```python
from build123d import *

# Parameters (mm, degrees)
SKETCH1_R           = 48.26
SKETCH1_R_2         = 26.56205
SKETCH1_W           = 81.370000074
SKETCH1_H           = 40
BOSS_EXTRUDE2_DEPTH = 15.24
SKETCH2_W           = 15.24
SKETCH2_H           = 24.76
BOSS_EXTRUDE3_DEPTH = 40
SKETCH3_R           = 3.9773733
SKETCH3_R_2         = 3.985133
CUT_EXTRUDE1_DEPTH  = 170.12215531
FILLET1_R           = 5.08
BOSS_EXTRUDE4_DEPTH = 66.04


with BuildPart() as part:
    # Sketch1 → Boss-Extrude2 (new body)
    # profile 1 of 2: a face of its own
    with BuildSketch(Plane(origin=(0, 0, 0), x_dir=(1, 0, 0), z_dir=(0, 1, 0))):
        Circle(SKETCH1_R)
        with Locations(Location((0, 0, 0), (0, 0, 90))):
            Circle(SKETCH1_R_2, mode=Mode.SUBTRACT)
    # profile 2 of 2: a face of its own
    with BuildSketch(Plane(origin=(0, 0, 0), x_dir=(1, 0, 0), z_dir=(0, 1, 0))):
        with Locations((83.372292456, 2.512722314)):
            Rectangle(SKETCH1_W, SKETCH1_H)
    extrude(amount=BOSS_EXTRUDE2_DEPTH)

    # Sketch2 → Boss-Extrude3 (add)
    with BuildSketch(Plane(origin=(0, 0, -22.512722314), x_dir=(-1, 0, 0), z_dir=(0, 0, -1))):
        with Locations((-116.437292493, 27.62)):
            Rectangle(SKETCH2_W, SKETCH2_H)
    extrude(amount=-BOSS_EXTRUDE3_DEPTH)

    # Sketch3 → Cut-Extrude1 (cut, through all)
    with BuildSketch(Plane.ZY.offset(-108.817292493)):
        with Locations((7.449197686, 31.22176)):
            Circle(SKETCH3_R)
        with Locations((-12.474642314, 31.22176)):
            Circle(SKETCH3_R_2)
    extrude(amount=-CUT_EXTRUDE1_DEPTH, mode=Mode.SUBTRACT)

    # Fillet1
    fillet1_edges = [part.edges().sort_by_distance(p)[0] for p in [
        (108.817292493, 15.24, -2.512722314),
    ]]
    fillet(fillet1_edges, radius=FILLET1_R)

    # Sketch5 → Boss-Extrude4 (add)
    with BuildSketch(Plane(origin=(0, 15.24, 0), x_dir=(1, 0, 0), z_dir=(0, 1, 0))):
        with BuildLine():
            ThreePointArc((0, 39.248127244), (39.248127244, 0), (0, -39.248127244))
            Line((0, -39.248127244), (-28.082238298, -39.248127244))
            ThreePointArc((-28.082238298, -39.248127244), (22.065570237, -42.920137583), (48.26, 0))
            ThreePointArc((48.26, 0), (22.065570237, 42.920137583), (-28.082238298, 39.248127244))
            Line((-28.082238298, 39.248127244), (0, 39.248127244))
        make_face()
    extrude(amount=BOSS_EXTRUDE4_DEPTH)


solid = part.part
```
CAD build for the part. Positions are in the model's coordinates, mm. A direction names the side the tool comes from. Round coordinates to 2 decimals unless told otherwise and drop trailing zeros. Loops run counter-clockwise (first coordinate to the right, second up) from the corner with the lowest first, then second, coordinate; pieces in that order, holes last. Notation, with made-up numbers: (76, 71.25) - (90, 71.25) arc R16 ccw to (90, 77.25) - close; hole circle Ø5 at (39.5, 49.5). An arc over 180 degrees is marked (long way). Return JSON: item names as keys, results as strings. Group by question number.
Q1. Band-saw the part on C-C on y = 50. Give the cut face in (x, z).
Q2. Band-saw the part on B-B on x = -2.5. Give the cut face in (y, z).
Q3. Tool access for faces 1 (the face through (116.331, 35.173, -12.993)), 2 (the face through (-14, 48, 39.248)), 3 (the face through (108.817, 30, -3)): list every direction of +Z, -Z, +X, -X, +Y, -Y with a clear straight run to the whole face (end or side of a thin tool).
Q4. Flat gauge pins, fed straight in: pin 1 Ø12 at (x, y) = (78.5, 11.5) entering from -Z; pin 2 Ø14 at (x, y) = (-17, 36) entering from +Z; pin 3 Ø20 at (x, z) = (74, 0) entering from +Y. Where does each tip first touch, or does it go through?
Q5. Two-plate mould, pull along Z, no slides. Class faces 4 (the face through (94, 11, 17.487)), 5 (the face through (37, 0, -1)), 6 (the face through (93, 11, -22.513)), 7 (the face through (116.3, 27.7, 9.3)): +Z half, -Z half, draft (parallel to the pull), parting line (faces both ways), or undercut.
Q6. Band-saw the part on D-D on y = 8. Give the cut face in (x, z).
Q7. Band-saw the part on A-A on y = 38. Give the cut face in (x, z), plus the area to 3 significant figures.
Q8. Drill centre lines: line 1 along X through (y, z) = (5, 0); line 2 along Y through (x, z) = (97, -9.5); line 3 along Z through (x, y) = (-15.5, 37). Where is each one in solid material? Low to high. Write a range as [from, to].
Solutions:
{
 "1": {"outline": "(-28.08, -39.25) arc R48.26 ccw (long way) to (-28.08, 39.25) - (0, 39.25) arc R39.25 cw to (0, -39.25) - close"},
 "2": {"outline": "(0, -48.2) - (81.28, -48.2) - (81.28, -39.25) - (15.24, -39.25) - (15.24, -26.44) - (0, -26.44) - close; (0, 26.44) - (15.24, 26.44) - (15.24, 39.25) - (81.28, 39.25) - (81.28, 48.2) - (0, 48.2) - close"},
 "3": {"face 1": "+X", "face 2": "-X, +Y", "face 3": "+Z, -Z, +Y"},
 "4": {"pin 1": "stops at z = -22.51", "pin 2": "stops at z = 47.21", "pin 3": "stops at y = 15.24"},
 "5": {"face 4": "+Z half", "face 5": "draft", "face 6": "-Z half", "face 7": "undercut"},
 "6": {"outline": "(42.69, -22.51) - (124.06, -22.51) - (124.06, 17.49) - (44.98, 17.49) arc R48.26 ccw (long way) to start; hole circle Ø53.12 at (0, 0)"},
 "7": {"outline": "(-28.08, -39.25) arc R48.26 ccw (long way) to (-28.08, 39.25) - (0, 39.25) arc R39.25 cw to (0, -39.25) - close; (108.82, -22.51) - (124.06, -22.51) - (124.06, 17.49) - (108.82, 17.49) - close", "area": "2,190 mm^2"},
 "8": {"line 1": "x = [-48.26, -26.56], [26.56, 124.06]", "line 2": "y = [0, 15.24]", "line 3": "z = [-45.7, -39.25], [39.25, 45.7]"}
}
